The model under review builds one solid part; all positions refer to its coordinate system, in mm. A direction names the side the tool comes from. Round coordinates to 2 decimals unless told otherwise and drop trailing zeros. Order: outer loops, then holes, each group sorted by start corner. A loop starts at its lowest first (then second) coordinate and runs counter-clockwise, first axis right, second up. Notation, with made-up numbers: M -15.5,-30.5 L -9.5,-30.5 A25 cw -9.5,-11.5 Z; hole C 36,12 d4. An arc over 180 degrees is marked long. Answer as a JSON object with one key per item and string values. Group by question number.
1) Consider section D-D, the plane y = 9.5. Write out the cut boundary in (x, z).
2) For faces 5 (the flat face through (-61.547, 70.588, -344.721)), 6 (the cylindrical face through (-77.45, 131.29, -477.92)), 7 (the flat face through (-13, 2.54, -154)), 8 (the flat face through (-89, 116.84, -474)), list the 3-axis set-ups (+Z, -Z, +X, -X, +Y, -Y) from which the entire face can be reached by the end or side of a thin tool; tool diameter is ignored.
3) Consider section A-A, the plane z = -457. Write out the cut boundary in (x, y), then the cut area to 3 significant figures.
4) Consider section C-C, the plane x = -58. Write out the cut boundary in (y, z), then the cut area to 3 significant figures.
5) To check wall thickness, follow line 1 (Y direction, x = -77, z = -482.6); line 2 (X direction, y = 137.9, z = -533.4) (3 decimals); line 3 (X direction, y = 139, z = -533). State the ranges of each line that lie inside material, in increasing order.
6) Consider section B-B, the plane y = 127. Write out the cut boundary in (x, z).
7) Insertion check: pin 1 Ø10 at (x, z) = (-88.9, -533.4) entering from -Y; pin 2 Ø22.5 at (y, z) = (124.5, -487) entering from +X; pin 3 Ø22.5 at (y, z) = (14.5, -155.5) entering from -X; pin 4 Ø22.5 at (x, z) = (-10, -80) entering from -Y. Each pin has a flat end and moves straight along its axis. Give the tip position at first contact, or say it passes through.
8) The part is to be moulded in two halves that separate along X. For faces 1 (the flat face through (-13, 22.86, -149)), 2 (the flat face through (0, 13, -155)), 3 (the flat face through (-99.06, 127, -469)), 4 (the flat face through (-25.4, 13, -151)), say which applies: +X half, -X half, draft (parallel to the pull), parting line (faces both ways), or undercut.
Autodesk Inventor part; units mm, degrees
ref_plane "YZ Plane" through (0, 0, 0) normal (1, 0, 0) x (0, 1, 0)
ref_plane "XZ Plane" through (0, 0, 0) normal (0, 1, 0) x (-1, 0, 0)
ref_plane "XY Plane" through (0, 0, 0) normal (0, 0, 1) x (1, 0, 0)
sketch "Sketch1" plane through (0, 0, 0) normal (0, 0, 1) x (1, 0, 0)
  line L0 (0, 0) -> (-25.4, 0)
  line L1 (-25.4, 0) -> (-25.4, 25.4)
  line L2 (-25.4, 25.4) -> (0, 25.4)
  line L3 (0, 25.4) -> (0, 0)
  line L4 (-2.54, 22.86) -> (-22.86, 22.86)
  line L5 (-22.86, 22.86) -> (-22.86, 2.54)
  line L6 (-22.86, 2.54) -> (-2.54, 2.54)
  line L7 (-2.54, 2.54) -> (-2.54, 22.86)
  dimension "d0" = 25.4
  dimension "d1" = 25.4
  dimension "d2" = 2.54
sketch "Sketch2" plane through (0, 0, 0) normal (1, 0, 0) x (0, 1, 0)
  line L0 (0, 0) -> (0, -304.8)
  line L1 (0, -304.8) -> (114.3, -406.4)
  line L2 (0, -304.8) -> (152.9283, -304.8) construction
  line L3 (114.3, -406.4) -> (114.3, -546.1)
  dimension "d3" = 304.8
  dimension "d5" = 139.7
  dimension "d6" = 114.3
  dimension "d7" = 101.6
sketch "Sketch3" plane through (0, 0, 0) normal (0, 1, 0) x (-1, 0, 0)
  line L0 (0, -406.4) -> (0, -546.1)
  line L1 (0, 0) -> (0, -304.8)
  line L2 (0, -304.8) -> (76.2, -406.4)
  line L3 (76.2, -406.4) -> (76.2, -546.1)
  dimension "d8" = 76.2
sketch3d "3D Sketch3"
  line L0 (0, 0, 0) -> (0, 0, -304.8)
  line L1 (0, 0, -304.8) -> (-76.2, 114.3, -406.4)
  line L2 (-76.2, 114.3, -406.4) -> (-76.2, 114.3, -546.1)
sweep "Sweep1" add profiles "Sketch1" path "3D Sketch3"
sketch "Sketch6" plane through (-76.2, 114.3, -546.1) normal (1, 0, 0) x (0, 0, -1)
  circle A0 centre (-63.5, 12.7) radius 6.35
  line L0 (0, 25.4) -> (0, 0)
  point P0 (-546.1, -114.3)
  dimension "d19" = 12.7
  dimension "d20" = 63.5
extrude "Extrusion3" cut sketch "Sketch6" against normal through all
sketch "Sketch7" plane through (-101.6, 139.7, -546.1) normal (0, 1, 0) x (1, 0, 0)
  circle A0 centre (12.7, -12.7) radius 3.175
  line L0 (0, -157.4592) -> (0, 0)
  line L1 (0, 0) -> (25.4, 0)
  point P0 (101.6, -546.1)
  dimension "d23" = 6.35
  dimension "d24" = 12.7
  dimension "d25" = 12.7
extrude "Extrusion4" cut sketch "Sketch7" against normal through all
properties part number "Arm 2"
Results list:
{
 "1": {"outline": "M -31.73,-306.14 L -6.33,-313.24 L 0,-300.81 L 0,0 L -2.54,0 L -2.54,-300.1 L -7.18,-309.21 L -27.5,-303.53 L -22.86,-294.42 L -22.86,0 L -25.4,0 L -25.4,-293.71 Z"},
 "2": {"face 5": "none", "face 6": "+X, -X", "face 7": "+Z", "face 8": "-Z"},
 "3": {"outline": "M -101.6,114.3 L -76.2,114.3 L -76.2,139.7 L -101.6,139.7 Z; hole M -99.06,116.84 L -78.74,116.84 L -78.74,137.16 L -99.06,137.16 Z", "area": "232 mm^2"},
 "4": {"outline": "M 48.9,-341.16 L 87,-382.13 L 112.4,-371.48 L 74.3,-330.51 Z; hole M 55.25,-344.19 L 85.73,-376.97 L 106.05,-368.45 L 75.57,-335.67 Z", "area": "521 mm^2"},
 "5": {"line 1": "114.3 to 120.65, 133.35 to 139.7", "line 2": "-101.6 to -92.075, -85.725 to -76.2", "line 3": "-101.6 to -92.05, -85.75 to -76.2"},
 "6": {"outline": "M -101.6,-546.1 L -99.06,-546.1 L -99.06,-488.95 L -101.6,-488.95 Z; M -101.6,-476.25 L -99.06,-476.25 L -99.06,-394.68 L -92.29,-381.39 L -71.97,-387.07 L -78.74,-400.36 L -78.74,-476.25 L -76.2,-476.25 L -76.2,-401.07 L -67.73,-384.46 L -93.13,-377.35 L -101.6,-393.97 Z; M -78.74,-546.1 L -76.2,-546.1 L -76.2,-488.95 L -78.74,-488.95 Z"},
 "7": {"pin 1": "y = 114.3", "pin 2": "x = -76.2", "pin 3": "x = -25.4", "pin 4": "y = 0"},
 "8": {"face 1": "undercut", "face 2": "+X half", "face 3": "undercut", "face 4": "-X half"}
}
